Source: CAD feature listing. Evaluate the final solid. Frame: model axes, mm. A direction names the side the tool comes from. Give positions to 0.01 mm unless a question says otherwise; leave off trailing zeros. Loops run counter-clockwise (first coordinate to the right, second up) from the corner with the lowest first, then second, coordinate; pieces in that order, holes last. Notation, with made-up numbers: (-24, 40.25) -> (-9, 40.25) arc R30 ccw to (-9, 71.25) -> close; hole circle Ø2 at (-20.5, 36.25). An arc over 180 degrees is marked (long way). Return JSON: item names as keys, results as strings. Group by question number.
(1) Cut plane A-A on x = 7. Return loops of the section in (y, z) (3 decimals).
(2) Cut plane B-B on z = 186. Return loops of the section in (x, y) (3 decimals), then the cut area to 3 significant figures.
(3) Draft query along X for faces 3 (the face through (22.225, 40, 326)), 4 (the face through (23.835, 36.109, 323.373)), 5 (the face through (0, 9, 326)), 6 (the face through (3.175, 41, 326)). Return one class per face: released by +X, released by -X, zero draft, split by the parting line, or undercut.
(4) Access query for faces 1 (the face through (2, 24, 0)), 2 (the face through (13, 3.175, 326)). Directions: +Z, -Z, +X, -X, +Y, -Y. A direction counts if a zero-diameter tool reaches every point of the face in a straight line with its end or side. Return the directions, or none.
(5) Ray query, line 1 (Y direction, x = 22.9, z = 330.2); line 2 (X direction, y = 45, z = 323.5) (3 decimals); line 3 (Y direction, x = 6.75, z = 94.5) (3 decimals). Return the intervals inside material, ascending. Write a range as from..to.
(6) Cut plane C-C on z = 330.2. Return loops of the section in (x, y) (3 decimals).
Autodesk Inventor part; units mm, degrees
ref_plane "YZ Plane" through (0, 0, 0) normal (1, 0, 0) x (0, 1, 0)
ref_plane "XZ Plane" through (0, 0, 0) normal (0, 1, 0) x (-1, 0, 0)
ref_plane "XY Plane" through (0, 0, 0) normal (0, 0, 1) x (1, 0, 0)
sketch "Sketch1" plane through (0, 0, 0) normal (0, 0, 1) x (1, 0, 0)
  line L0 (0, 0) -> (25.4, 0)
  line L1 (25.4, 0) -> (25.4, 50.8)
  line L2 (25.4, 50.8) -> (0, 50.8)
  line L3 (0, 50.8) -> (0, 0)
  line L4 (3.175, 3.175) -> (22.225, 3.175)
  line L5 (22.225, 3.175) -> (22.225, 47.625)
  line L6 (22.225, 47.625) -> (3.175, 47.625)
  line L7 (3.175, 47.625) -> (3.175, 3.175)
  dimension "d0" = 25.4
  dimension "d1" = 50.8
  dimension "d2" = 19.05
  dimension "d3" = 44.45
  dimension "d4" = 3.175
  dimension "d5" = 3.175
extrude "Extrusion1" add sketch "Sketch1" along normal blind 660.4
sketch "Sketch2" plane through (25.4, 0, 0) normal (1, 0, 0) x (0, 0, -1)
  line L0 (0, 0) -> (0, 50.8)
  line L1 (0, 50.8) -> (-660.4, 50.8)
  line L2 (-660.4, 0) -> (-660.4, 50.8)
  line L3 (0, 0) -> (-660.4, 0)
  circle A0 centre (-330.2, 25.4) radius 12.7
  line L4 (-603.25, 25.4) -> (-603.25, 20.6375) construction
  line L5 (-603.25, 20.6375) -> (-603.25, 30.1625) construction
  line L6 (-577.85, 25.4) -> (-577.85, 20.6375) construction
  line L7 (-577.85, 20.6375) -> (-577.85, 30.1625) construction
  line L8 (-82.55, 25.4) -> (-82.55, 20.6375) construction
  line L9 (-82.55, 25.4) -> (-77.7875, 25.4) construction
  line L10 (-82.55, 20.6375) -> (-82.55, 30.1625) construction
  line L11 (-57.15, 25.4) -> (-57.15, 20.6375) construction
  line L12 (-57.15, 25.4) -> (-52.3875, 25.4) construction
  line L13 (-57.15, 20.6375) -> (-57.15, 30.1625) construction
  arc A1 (-603.25, 30.1625) -> (-603.25, 20.6375) centre (-603.047, 25.4) ccw
  arc A2 (-577.85, 20.6375) -> (-577.85, 30.1625) centre (-577.2085, 25.4) ccw
  arc A3 (-82.55, 30.1625) -> (-82.55, 20.6375) centre (-81.7597, 25.4) ccw
  arc A4 (-57.15, 20.6375) -> (-57.15, 30.1625) centre (-57.2051, 25.4) ccw
  line L14 (-82.55, 30.1625) -> (-57.15, 30.1625)
  line L15 (-57.15, 20.6375) -> (-82.55, 20.6375)
  line L16 (-603.25, 30.1625) -> (-577.85, 30.1625)
  line L17 (-577.85, 20.6375) -> (-603.25, 20.6375)
  dimension "d8" = 25.4
  dimension "d9" = 330.2
  dimension "d10" = 25.4
  dimension "d11" = 25.4
  dimension "d12" = 25.4
  dimension "d13" = 25.4
  dimension "d14" = 25.4
  dimension "d15" = 57.15
  dimension "d16" = 57.15
  dimension "d17" = 82.55
  dimension "d18" = 82.55
  dimension "d19" = 4.7625
  dimension "d20" = 9.525
  dimension "d21" = 4.7625
  dimension "d22" = 9.525
  dimension "d23" = 4.7625
  dimension "d24" = 90
  dimension "d25" = 9.525
  dimension "d26" = 4.7625
  dimension "d27" = 90
  dimension "d28" = 9.525
  dimension "d29" = 4.7668
  dimension "d30" = 4.8055
  dimension "d31" = 4.8276
  dimension "d32" = 4.7628
extrude "Extrusion2" cut sketch "Sketch2" against normal blind 762 contours A0 | L16 A2 L17 A1 | L14 A4 L15 A3
properties part number "frame_long"
Answers:
{
 "1": {"outline": "(0, 0) -> (3.175, 0) -> (3.175, 660.4) -> (0, 660.4) -> close; (47.625, 0) -> (50.8, 0) -> (50.8, 660.4) -> (47.625, 660.4) -> close"},
 "2": {"outline": "(0, 0) -> (25.4, 0) -> (25.4, 50.8) -> (0, 50.8) -> close; hole (3.175, 3.175) -> (22.225, 3.175) -> (22.225, 47.625) -> (3.175, 47.625) -> close", "area": "444 mm²"},
 "3": {"face 3": "undercut", "face 4": "zero draft", "face 5": "released by -X", "face 6": "undercut"},
 "4": {"face 1": "-Z, +X, -X, +Y, -Y", "face 2": "+Z, -Z"},
 "5": {"line 1": "0..12.7, 38.1..50.8", "line 2": "0..3.175, 22.225..25.4", "line 3": "0..3.175, 47.625..50.8"},
 "6": {"outline": "(0, 0) -> (25.4, 0) -> (25.4, 12.7) -> (22.225, 12.7) -> (22.225, 3.175) -> (3.175, 3.175) -> (3.175, 12.7) -> (0, 12.7) -> close; (0, 38.1) -> (3.175, 38.1) -> (3.175, 47.625) -> (22.225, 47.625) -> (22.225, 38.1) -> (25.4, 38.1) -> (25.4, 50.8) -> (0, 50.8) -> close"}
}
